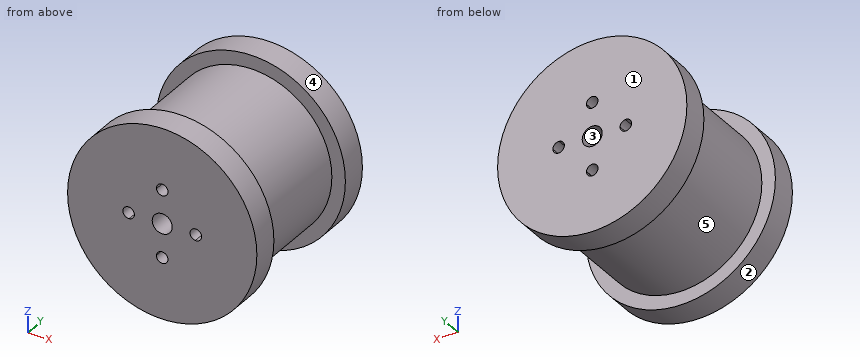
```python
from build123d import *

# Parameters (mm, degrees)
F0_R          = 19.05
F1_DEPTH      = 13.335
F1_DEPTH_BACK = 13.335
F2_R          = 22.225
F3_DEPTH      = 6.35
F4_R          = 22.225
F5_DEPTH      = 6.35
F6_R          = 2.3495
F7_DEPTH      = 39.37


with BuildPart() as f1:
    # F0 (on Front) → F1 (new body, two sides)
    with BuildSketch(Plane.XZ) as f1_sk:
        Circle(F0_R)
    extrude(amount=F1_DEPTH)
    extrude(f1_sk.sketch, amount=-F1_DEPTH_BACK)

    # F2 (on face) → F3 (join)
    with BuildSketch(Plane.XZ.offset(13.335)):
        Circle(F2_R)
    extrude(amount=F3_DEPTH)

    # F4 (on face) → F5 (join)
    with BuildSketch(Plane(origin=(0, 13.335, 0), x_dir=(-1, 0, 0), z_dir=(0, 1, 0))):
        Circle(F4_R)
    extrude(amount=F5_DEPTH)

    # F6 (on face) → F7 (cut)
    with BuildSketch(Plane.XZ.offset(19.685)):
        with BuildLine():
            ThreePointArc((-6.53415, 0), (-6.8901410167, 0.9144734525), (-7.770720471, 1.3475682734))
            ThreePointArc((-7.770720471, 1.3475682734), (-7.8867, 0), (-7.770720471, -1.3475682734))
            ThreePointArc((-7.770720471, -1.3475682734), (-6.8901410167, -0.9144734525), (-6.53415, 0))
        make_face()
        with BuildLine():
            ThreePointArc((-7.770720471, -1.3475682734), (-7.8867, 0), (-7.770720471, 1.3475682734))
            ThreePointArc((-7.770720471, 1.3475682734), (-9.23925, 0), (-7.770720471, -1.3475682734))
        make_face()
        with BuildLine():
            ThreePointArc((7.770720471, -1.3475682734), (7.8576516221, -0.676275), (7.8867, 0))
            ThreePointArc((7.8867, 0), (7.8576516221, 0.676275), (7.770720471, 1.3475682734))
            ThreePointArc((7.770720471, 1.3475682734), (6.53415, 0), (7.770720471, -1.3475682734))
        make_face()
        with BuildLine():
            ThreePointArc((7.770720471, 1.3475682734), (7.8576516221, 0.676275), (7.8867, 0))
            ThreePointArc((7.8867, 0), (7.8576516221, -0.676275), (7.770720471, -1.3475682734))
            ThreePointArc((7.770720471, -1.3475682734), (8.8011734525, -0.9965589833), (9.23925, 0))
            ThreePointArc((9.23925, 0), (8.8011734525, 0.9965589833), (7.770720471, 1.3475682734))
        make_face()
        Circle(F6_R)
        with BuildLine():
            ThreePointArc((-1.3475682734, -7.770720471), (0, -7.8867), (1.3475682734, -7.770720471))
            ThreePointArc((1.3475682734, -7.770720471), (0, -6.53415), (-1.3475682734, -7.770720471))
        make_face()
        with BuildLine():
            ThreePointArc((1.35255, -7.8867), (1.3513039944, -7.8286567645), (1.3475682734, -7.770720471))
            ThreePointArc((1.3475682734, -7.770720471), (0, -7.8867), (-1.3475682734, -7.770720471))
            ThreePointArc((-1.3475682734, -7.770720471), (-0.0580432355, -9.2380039944), (1.35255, -7.8867))
        make_face()
        with BuildLine():
            ThreePointArc((-1.3475682734, 7.770720471), (0, 6.53415), (1.3475682734, 7.770720471))
            ThreePointArc((1.3475682734, 7.770720471), (0, 7.8867), (-1.3475682734, 7.770720471))
        make_face()
        with BuildLine():
            ThreePointArc((-1.3475682734, 7.770720471), (0, 7.8867), (1.3475682734, 7.770720471))
            ThreePointArc((1.3475682734, 7.770720471), (1.3513039944, 7.8286567645), (1.35255, 7.8867))
            ThreePointArc((1.35255, 7.8867), (-0.0580432355, 9.2380039944), (-1.3475682734, 7.770720471))
        make_face()
    extrude(amount=-F7_DEPTH, mode=Mode.SUBTRACT)


solid = f1.part
```
The listing builds one solid part. Answer for the finished solid, in the listing's coordinates (mm). Face numbers are marked on the shaded views. A direction names the side the tool comes from. Give positions to 0.01 mm unless a question says otherwise; leave off trailing zeros. Order: outer loops, then holes, each group sorted by start corner. A loop starts at its lowest first (then second) coordinate and runs counter-clockwise, first axis right, second up. Notation, with made-up numbers: (6.25, -0.75) - (64.25, -0.75) arc R24 cw to (64.25, 30.25) - close; hole circle Ø1 at (-32, 69). An arc over 180 degrees is marked (long way). Answer in a Markdown table with one row per item. Add a question column.
Q1. The part is cut by section D-D (z = -13). Determine the outline of the cut face in (x, y) (3 decimals), then the cut area to 3 significant figures.
Q2. The part is cut by section C-C (x = 8.5). Determine the outline of the cut face in (y, z) (3 decimals), then the cut area to 3 significant figures.
Q3. Find the intervals of material crossed by line 1 along Z through (x, y) = (0, -4); line 2 along X through (y, z) = (6.5, 1); line 3 along Z through (x, y) = (-2, 11), in increasing order. Write a range as [from, to].
Q4. The part is cut by section B-B (y = -3.5). Determine the outline of the cut face in (x, z), then the cut area to 3 significant figures.
Q5. For a pull along X with two mould halves and no side action, classify the marked faces 1, 2 and 3 as released by +X, released by -X, zero draft, split by the parting line, or undercut.
Q6. The part is cut by section A-A (x = 0). Give the number of separate pieces and of enclosed holes in the cut face, then the cut area to 3 significant figures.
Q7. Which of the six approach directions +Z, -Z, +X, -X, +Y, -Y give full straight-line access (tool end or side, diameter ignored) to the marked faces 4 and 5?
Q8. Given P1, Ø3, axis at x = -5, y = -8.5, coming from the +Z side; P2, Ø5, axis at x = 1.5, y = 9, coming from the -Z side; P3, Ø6, axis at x = -12.5, y = 4.5, coming from the -Z side, each flat-ended and moving along its own axis, determine where each tip first touches the part or whether it passes through.
Determined:
| question | item | result |
|---|---|---|
| 1 | outline | (-18.026, -19.685) - (18.026, -19.685) - (18.026, -13.335) - (13.925, -13.335) - (13.925, 13.335) - (18.026, 13.335) - (18.026, 19.685) - (-18.026, 19.685) - (-18.026, 13.335) - (-13.925, 13.335) - (-13.925, -13.335) - (-18.026, -13.335) - close |
| 1 | area | 1,200 mm² |
| 2 | outline | (-19.685, -20.535) - (-13.335, -20.535) - (-13.335, -17.049) - (13.335, -17.049) - (13.335, -20.535) - (19.685, -20.535) - (19.685, -1.206) - (-19.685, -1.206) - close; (-19.685, 1.206) - (19.685, 1.206) - (19.685, 20.535) - (13.335, 20.535) - (13.335, 17.049) - (-13.335, 17.049) - (-13.335, 20.535) - (-19.685, 20.535) - close |
| 2 | area | 1,340 mm² |
| 3 | line 1 | z = [-19.05, -9.24], [-6.53, -2.35], [2.35, 6.53], [9.24, 19.05] |
| 3 | line 2 | x = [-19.02, -8.8], [-6.98, -2.13], [2.13, 6.98], [8.8, 19.02] |
| 3 | line 3 | z = [-18.94, -1.23], [1.23, 18.94] |
| 4 | outline | circle Ø38.1 at (0, 0); hole circle Ø2.71 at (-7.89, 0); hole circle Ø4.7 at (0, 0); hole circle Ø2.71 at (0, -7.89); hole circle Ø2.71 at (0, 7.89); hole circle Ø2.71 at (7.89, 0) |
| 4 | area | 1,100 mm² |
| 5 | face 1 | zero draft |
| 5 | face 2 | split by the parting line |
| 5 | face 3 | undercut |
| 6 | separate pieces | 4 |
| 6 | enclosed holes | 0 |
| 6 | area | 1,180 mm² |
| 7 | face 4 | +Y, -Y |
| 7 | face 5 | none |
| 8 | P1 | stops at z = 18.73 |
| 8 | P2 | stops at z = -19.05 |
| 8 | P3 | stops at z = -16.51 |
